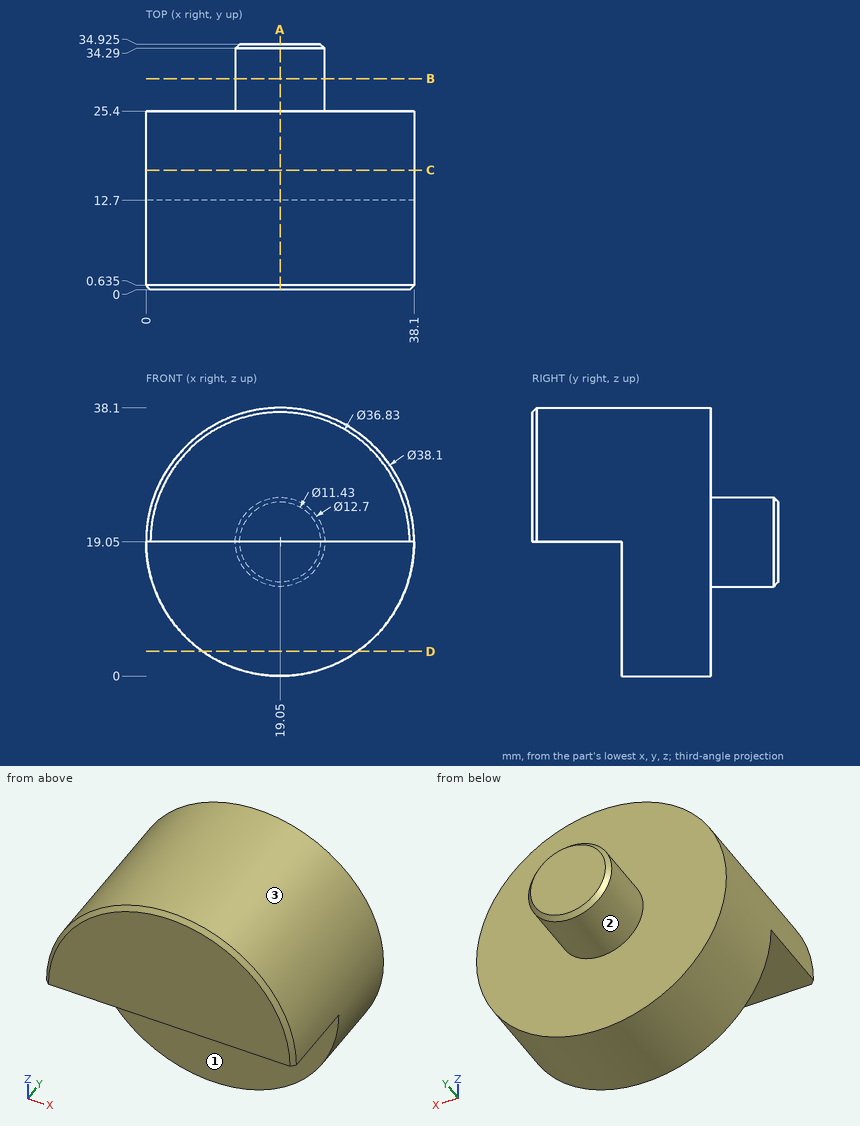
For this review, use the dimensioned drawing (mm, ordinates from the lowest corner) and the shaded views. A direction names the side the tool comes from. Give positions to 0.01 mm unless a question says otherwise; leave off trailing zeros. Order: outer loops, then holes, each group sorted by start corner. A loop starts at its lowest first (then second) coordinate and runs counter-clockwise, first axis right, second up. Notation, with made-up numbers: (61, 83) - (68, 83) arc R15 ccw to (68, 102) - close; hole circle Ø3 at (58, 46). An arc over 180 degrees is marked (long way). Use CSV: the item, a comma, the result in double quotes. Start each with the question number.
Q1. We need section B-B, the plane y = 30. Write out the cut boundary in (x, z), and give its area (3 significant figures).
Q2. To check wall thickness, follow line 1 along Y through (x, z) = (33, 13); line 2 along Z through (x, y) = (18.5, 16); line 3 along Y through (x, z) = (27.5, 26). State the ranges of each line that lie inside material, in increasing order. Write a range as [from, to].
Q3. Tool access review of the marked faces 1, 2 and 3: name each direction out of +Z, -Z, +X, -X, +Y, -Y from which nothing blocks a thin tool from reaching the whole face with its end or side.
Q4. We need section A-A, the plane x = 19.05. Write out the cut boundary in (y, z) (3 decimals).
Q5. We need section D-D, the plane z = 3.5. Write out the cut boundary in (x, y), and give its area (3 significant figures).
Q6. Clearance check with flat-ended pins moving along their axes: pin 1 Ø10 at (y, z) = (17, 25) entering from -X; pin 2 Ø2 at (x, z) = (16, 6.5) entering from +Y; pin 3 Ø6.5 at (x, y) = (21.5, 7.5) entering from -Z. State where each tip first meets the part, or that it passes through.
Q7. We need section C-C, the plane y = 17. Write out the cut boundary in (x, z), and give its area (3 significant figures).
Outcome:
1,outline,"circle Ø12.7 at (19.05, 19.05)"
1,area,"127 mm^2"
2,line 1,"y = [12.7, 25.4]"
2,line 2,"z = [0.01, 38.09]"
2,line 3,"y = [0, 25.4]"
3,face 1,"-Z, +X, -X, -Y"
3,face 2,"+Y"
3,face 3,"+Y, -Y"
4,outline,"(0, 19.05) - (12.7, 19.05) - (12.7, 0) - (25.4, 0) - (25.4, 12.7) - (34.29, 12.7) - (34.925, 13.335) - (34.925, 24.765) - (34.29, 25.4) - (25.4, 25.4) - (25.4, 38.1) - (0.635, 38.1) - (0, 37.465) - close"
5,outline,"(8.05, 12.7) - (30.05, 12.7) - (30.05, 25.4) - (8.05, 25.4) - close"
5,area,"280 mm^2"
6,pin 1,"stops at x = 0.02"
6,pin 2,"stops at y = 25.4"
6,pin 3,"stops at z = 19.05"
7,outline,"circle Ø38.1 at (19.05, 19.05)"
7,area,"1,140 mm^2"
